Autodesk Inventor part; units mm, degrees
ref_plane "YZ Plane" through (0, 0, 0) normal (1, 0, 0) x (0, 1, 0)
ref_plane "XZ Plane" through (0, 0, 0) normal (0, 1, 0) x (-1, 0, 0)
ref_plane "XY Plane" through (0, 0, 0) normal (0, 0, 1) x (1, 0, 0)
sketch "Sketch1" plane through (0, 0, 0) normal (0, 0, 1) x (1, 0, 0)
  circle A0 centre (0, 0) radius 2.5
  dimension "d0" = 5
extrude "Extrusion1" add sketch "Sketch1" along normal blind 5
sketch "Sketch2" plane through (0, 0, 5) normal (0, 0, 1) x (1, 0, 0)
  circle A0 centre (0, 0) radius 2.2
  circle A1 centre (0, 0) radius 2.5
  circle A2 centre (0, 0) radius 2
  dimension "d3" = 4.4
  dimension "d4" = 4
extrude "Extrusion2" add sketch "Sketch2" along normal blind 10 contours A0
sketch "Sketch3" plane through (0, 0, 5) normal (0, 0, 1) x (1, 0, 0)
  circle A0 centre (0, 0) radius 0.15
  dimension "d7" = 0.3
extrude "Extrusion3" add sketch "Sketch3" along normal blind 10
sketch "Sketch4" plane through (0, 0, 15) normal (0, 0, 1) x (1, 0, 0)
  circle A0 centre (0, 0) radius 2.5
extrude "Extrusion4" add sketch "Sketch4" along normal blind 5
properties part number "EuropeanFuse3A"
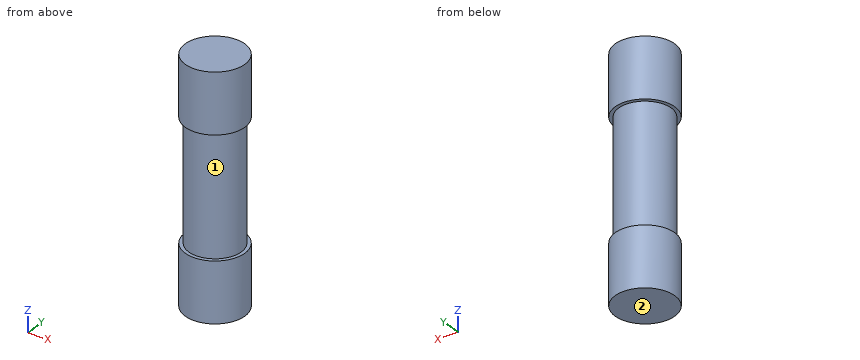
Input: part model. Units: mm. Frame: model coordinates. Face numbers are marked on the shaded views. A direction names the side the tool comes from. Coordinates: 2 decimals unless noted, no trailing zeros. Loops run counter-clockwise (first coordinate to the right, second up) from the corner with the lowest first, then second, coordinate; pieces in that order, holes last. Notation, with made-up numbers: M -28,13 L -19,13 A12 ccw -19,20 Z; hole C -6,22.25 d8. An arc over 180 degrees is marked long. Answer in a Markdown table with one row per item.
1. Material intervals for line 1 (Y direction, x = 0, z = 8.5); line 2 (Z direction, x = -0.3, y = 0.75); line 3 (X direction, y = 0.1, z = 8.5), sorted ascending.
Response:
| item | result |
|---|---|
| line 1 | y = -2.2 to -2, -0.15 to 0.15, 2 to 2.2 |
| line 2 | z = 0 to 5, 15 to 20 |
| line 3 | x = -2.2 to -2, -0.11 to 0.11, 2 to 2.2 |
2. Reachability of the marked faces 1 and 2 from +Z, -Z, +X, -X, +Y, -Y: full face, straight path, thin tool, end or side. Return the list, or none.
Response:
| item | result |
|---|---|
| face 1 | none |
| face 2 | -Z, +X, -X, +Y, -Y |
3. Section B-B, the plane z = 7. Output: boundary loops of the cut face in (x, y).
Response:
| item | result |
|---|---|
| outline | C 0,0 d4.4; C 0,0 d0.3; hole C 0,0 d4 |
4. Section D-D, the plane z = 1.5. Output: boundary loops of the cut face in (x, y), then the cut area to 3 significant figures.
Response:
| item | result |
|---|---|
| outline | C 0,0 d5 |
| area | 19.6 mm2 |
5. First-contact query: pin 1 (1 mm diameter, centred on x = 2, z = 4, fed in from +Y). Flat tip, straight axial feed; report the tip coordinate or a pass-through.
Response:
| item | result |
|---|---|
| pin 1 | stops at y = 2 |
6. Section C-C, the plane y = 0.8. Output: boundary loops of the cut face in (x, z).
Response:
| item | result |
|---|---|
| outline | M -2.37,0 L 2.37,0 L 2.37,5 L 2.05,5 L 2.05,15 L 2.37,15 L 2.37,20 L -2.37,20 L -2.37,15 L -2.05,15 L -2.05,5 L -2.37,5 Z; hole M -1.83,5 L 1.83,5 L 1.83,15 L -1.83,15 Z |
7. Section A-A, the plane x = -1.15. Output: boundary loops of the cut face in (y, z), then the cut area to 3 significant figures.
Response:
| item | result |
|---|---|
| outline | M -2.22,0 L 2.22,0 L 2.22,5 L 1.88,5 L 1.88,15 L 2.22,15 L 2.22,20 L -2.22,20 L -2.22,15 L -1.88,15 L -1.88,5 L -2.22,5 Z; hole M -1.64,5 L 1.64,5 L 1.64,15 L -1.64,15 Z |
| area | 49.2 mm2 |
